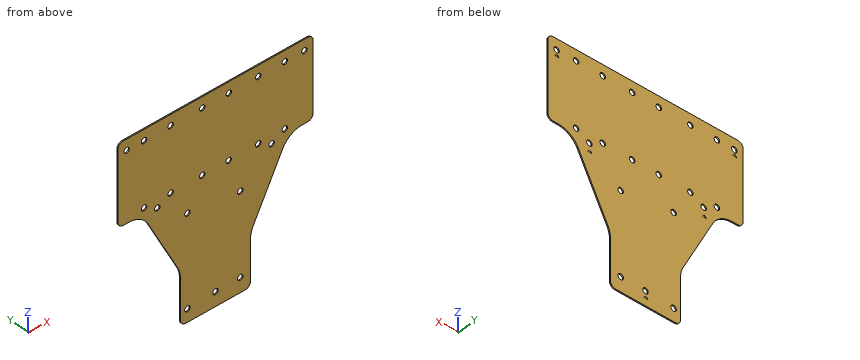
```python
from build123d import *

# Parameters (mm, degrees)
F0_W     = 178
F0_H     = 188
F1_DEPTH = 1
F2_R     = 2.5
F3_DEPTH = 1.001
F5_DEPTH = 1.001
F6_R     = 5
F7_R     = 20
F9_DEPTH = 0.3


with BuildPart() as f1:
    # F0 (on Front) → F1 (new body)
    with BuildSketch(Plane.XZ):
        with Locations((0, -11)):
            Rectangle(F0_W, F0_H)
    extrude(amount=F1_DEPTH)

    # F2 (on face) → F3 (cut, through all)
    with BuildSketch(Plane(origin=(0, 0, 0), x_dir=(-1, 0, 0), z_dir=(0, 1, 0))):
        with Locations((-81, 73.2)):
            Circle(F2_R)
        with Locations((81, 73.2)):
            Circle(F2_R)
        with Locations((53, 8.5)):
            Circle(F2_R)
        with Locations((-51.1, 8.5)):
            Circle(F2_R)
        with Locations((0, -92)):
            Circle(F2_R)
        with Locations((-22.6, -91.8)):
            Circle(F2_R)
        with Locations((25.6, -93.3)):
            Circle(F2_R)
        with Locations((-22.6, -17.2)):
            Circle(F2_R)
        with Locations((25.6, -10.6)):
            Circle(F2_R)
        with Locations((-63.2, 73.2)):
            Circle(F2_R)
        with Locations((-39, 73.2)):
            Circle(F2_R)
        with Locations((-39, 15)):
            Circle(F2_R)
        with Locations((-63.2, 15)):
            Circle(F2_R)
        with Locations((40.9, 73.2)):
            Circle(F2_R)
        with Locations((65.1, 73.2)):
            Circle(F2_R)
        with Locations((65.1, 15)):
            Circle(F2_R)
        with Locations((40.9, 15)):
            Circle(F2_R)
        with Locations((-12.1, 73.2)):
            Circle(F2_R)
        with Locations((12.1, 73.2)):
            Circle(F2_R)
        with Locations((-12.1, 15)):
            Circle(F2_R)
        with Locations((12.1, 15)):
            Circle(F2_R)
    extrude(amount=-F3_DEPTH, mode=Mode.SUBTRACT)

    # F4 (on face) → F5 (cut, through all)
    with BuildSketch(Plane(origin=(0, 0, 0), x_dir=(-1, 0, 0), z_dir=(0, 1, 0))):
        Polygon((-94, -113), (-32, -113), (-32, -58), (-67, 10), (-94, 10), align=None)
        Polygon((32, -58), (32, -113), (94, -113), (94, 10), (67, 10), align=None)
    extrude(amount=-F5_DEPTH, mode=Mode.SUBTRACT)

    # F6
    f6_edges = [f1.edges().sort_by_distance(p)[0] for p in [
        (89, -0.5, 83),
        (-89, -0.5, 83),
        (-89, -0.5, 10),
        (-32, -0.5, -105),
        (32, -0.5, -105),
        (89, -0.5, 10),
    ]]
    fillet(f6_edges, radius=F6_R)

    # F7
    f7_edges = [f1.edges().sort_by_distance(p)[0] for p in [
        (67, -0.5, 10),
        (32, -0.5, -58),
        (-32, -0.5, -58),
        (-67, -0.5, 10),
    ]]
    fillet(f7_edges, radius=F7_R)

    # F8 (on face) → F9 (cut)
    with BuildSketch(Plane.XZ):
        Polygon((82.946427, 67.366861), (80.661148, 69.433466), (78.453593, 67.366861), align=None)
        Polygon((52.970854, 0.529755), (50.685575, 2.59636), (48.47802, 0.529755), align=None)
        Polygon((-51.300323, -0.06174), (-53.585603, 2.004865), (-55.793157, -0.06174), align=None)
        Polygon((1.892914, -98.51862), (-0.392365, -96.452015), (-2.59992, -98.51862), align=None)
        Polygon((-78.801448, 67.370405), (-81.086727, 69.43701), (-83.294282, 67.370405), align=None)
    extrude(amount=F9_DEPTH, mode=Mode.SUBTRACT)


solid = f1.part
```
Part model, mm, in its own coordinate system. Round coordinates to 2 decimals unless told otherwise and drop trailing zeros. Loops run counter-clockwise (first coordinate to the right, second up) from the corner with the lowest first, then second, coordinate; pieces in that order, holes last. Notation, with made-up numbers: (53.25, -17.5) -> (74.25, -17.5) arc R14 cw to (74.25, -5.5) -> close; hole circle Ø7 at (-38.5, 35.5). An arc over 180 degrees is marked (long way). Use one line per item in the form item = value. Start each with the question number.
Item 1: Band-saw the part on A-A (z = -17.2). List the corners of the cut face in (x, y).
Item 2: Drop a flat-ended pin along its axis: pin 1 Ø1 at (x, z) = (-82, 68.5) entering from +Y. Give the stop position or say it passes through.
Item 3: Band-saw the part on B-B (x = -12.1). List the corners of the cut face in (y, z).
Item 4: Drill centre lines: line 1 along Z through (x, y) = (-12.1, -0.75); line 2 along Z through (x, y) = (-65.1, -0.25); line 3 along Z through (x, y) = (81, -0.45). Where is each one in solid material? Low to high.
Item 5: Band-saw the part on D-D (y = -0.5). Give the number of separate pieces and of enclosed holes in the cut face, plus the area to 3 significant figures.
Item 6: Band-saw the part on C-C (z = -74.5). List the corners of the cut face in (x, y).
Data:
q1.outline = (-53, -1) -> (20.1, -1) -> (20.1, 0) -> (-53, 0) -> close; (25.1, -1) -> (53, -1) -> (53, 0) -> (25.1, 0) -> close
q2.pin_1 = 0
q3.outline = (-1, -105) -> (0, -105) -> (0, 12.5) -> (-1, 12.5) -> close; (-1, 17.5) -> (0, 17.5) -> (0, 70.7) -> (-1, 70.7) -> close; (-1, 75.7) -> (0, 75.7) -> (0, 83) -> (-1, 83) -> close
q4.line_1 = -105 to 12.5, 17.5 to 70.7, 75.7 to 83
q4.line_2 = 4.18 to 12.5, 17.5 to 70.7, 75.7 to 83
q4.line_3 = 10 to 70.7, 75.7 to 83
q5.separate_pieces = 1
q5.enclosed_holes = 21
q5.area = 22,300 mm^2
q6.outline = (-32, -1) -> (32, -1) -> (32, 0) -> (-32, 0) -> close
